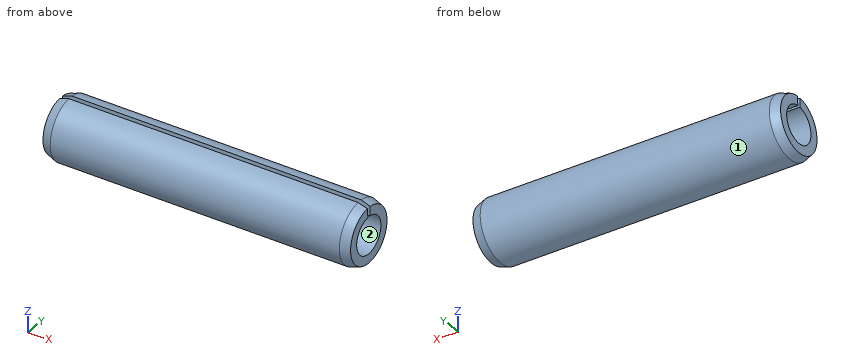
```python
from build123d import *

# Parameters (mm, degrees)
GAP_DEPTH = 11.099504938


with BuildPart() as part:
    # BodySke → Body (revolve)
    with BuildSketch(Plane.XY, mode=Mode.PRIVATE) as body_sk:
        Polygon((0, 0.6), (10, 0.6), (10, 0.9), (9.7, 1), (0.3, 1), (0, 0.9), align=None)
    revolve(body_sk.sketch.rotate(Axis((-9.525, 0, 0), (1, 0, 0)), 90), axis=Axis((-9.525, 0, 0), (1, 0, 0)))

    # GapSke → Gap (cut, through all)
    with BuildSketch(Plane(origin=(0, 0, 0), x_dir=(0, -1, 0), z_dir=(-1, 0, 0))):
        with BuildLine():
            Line((0, 0), (0.080028278, 1.01685568))
            ThreePointArc((0.080028278, 1.01685568), (0, 1.02), (-0.080028278, 1.01685568))
            Line((-0.080028278, 1.01685568), (0, 0))
        make_face()
    extrude(amount=-GAP_DEPTH, mode=Mode.SUBTRACT)


solid = part.part
```
The model under review builds one solid part; all positions refer to its coordinate system, in mm. Face numbers are marked on the shaded views. Round coordinates to 2 decimals unless told otherwise and drop trailing zeros. Loops run counter-clockwise (first coordinate to the right, second up) from the corner with the lowest first, then second, coordinate; pieces in that order, holes last. Notation, with made-up numbers: M 65.5,59 L 83.5,59 A15 ccw 83.5,72 Z; hole C 45,-23 d1. An arc over 180 degrees is marked long. Answer as a JSON object with one key per item and string values.
(1) Draft analysis for pull direction Y (two halves, no side actions). For the marked faces 1 and 2, state which applies: released by +Y, released by -Y, zero draft, split by the parting line, or undercut.
Resolved:
{"face 1": "split by the parting line", "face 2": "undercut"}
(2) To check wall thickness, follow line 1 along Y through (x, z) = (2.5, 0); line 2 along Z through (x, y) = (7.75, 0); line 3 along Z through (x, y) = (3.75, 0.4). State the ranges of each line that lie inside material, in increasing order.
Resolved:
{"line 1": "-1 to -0.6, 0.6 to 1", "line 2": "-1 to -0.6", "line 3": "-0.92 to -0.45, 0.45 to 0.92"}
(3) Take a section at B-B on x = 5. Give the boundary of the cut face in (y, z).
Resolved:
{"outline": "M -0.08,1 A1 ccw long 0.08,1 L 0.05,0.6 A0.6 cw long -0.05,0.6 Z"}
(4) Take a section at A-A on z = 0. Give the boundary of the cut face in (x, y).
Resolved:
{"outline": "M 0,-0.9 L 0.3,-1 L 9.7,-1 L 10,-0.9 L 10,-0.6 L 0,-0.6 Z; M 0,0.6 L 10,0.6 L 10,0.9 L 9.7,1 L 0.3,1 L 0,0.9 Z"}
